Geometry: final body of the model. Coordinates: model frame, mm. Face numbers are marked on the shaded views. Round coordinates to 2 decimals unless told otherwise and drop trailing zeros. Order: outer loops, then holes, each group sorted by start corner. A loop starts at its lowest first (then second) coordinate and runs counter-clockwise, first axis right, second up. Notation, with made-up numbers: (54, 56.5) -> (65, 56.5) arc R7 ccw to (65, 63.5) -> close; hole circle Ø6 at (54, -2). An arc over 180 degrees is marked (long way). Put each result on its own line as item: value.
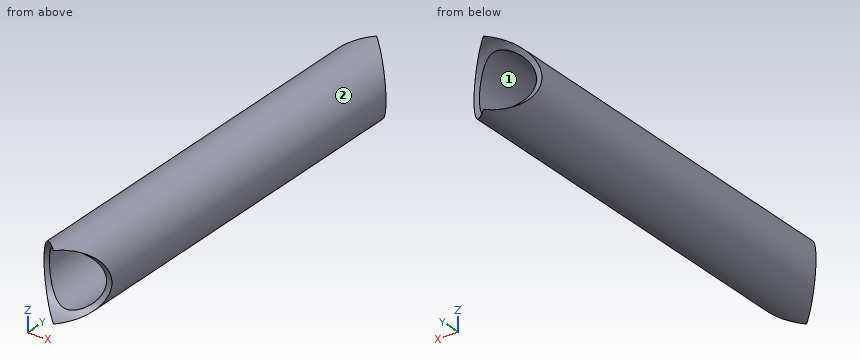
Solid Edge part; units mm, degrees
sketch "Sketch1" plane through (0, 0, 0) normal (0, 0, 1) x (1, 0, 0)
  line L0 (0, 0) -> (0, 164)
sketch "Sketch2" plane through (0, 0, 0) normal (0, -1, 0) x (1, 0, 0)
  circle A0 centre (0, 0) radius 12.5
sweep "SweptProtrusion_1" add profiles "Sketch2" path "Sketch1"
shell "Thinwall_1" thickness 2 removed faces 2 at (-8.0833, 0, 8.5833) at (-8.0833, 164, 8.5833)
sketch "Sketch3" plane through (0, 0, 0) normal (1, 0, 0) x (0, 1, 0)
  circle A0 centre (0, 0) radius 12.5
  circle A1 centre (164, 0) radius 12.5
extrude "Cutout1" cut sketch "Sketch3" along normal through all and the other way through all
properties material "Stainless steel"
1. Draft query along X for the marked faces 1 and 2. Return one class per face: +X half, -X half, draft (parallel to the pull), parting line (faces both ways), or undercut.
Ans:
face 1: undercut
face 2: parting line
2. Contact query for flat-ended pins moving along their axis: P1, Ø2, axis at y = 81, z = 4, coming from the -X side; P2, Ø5, axis at x = -6, y = 57, coming from the -Z side; P3, Ø3, axis at y = 21, z = -7, coming from the -X side (3 decimals). Output: stop coordinate, or through.
Ans:
P1: x = -12.13
P2: z = -12
P3: x = -11.225
3. Cut plane B-B on z = 0. Return loops of the section in (x, y), and give its area (3 significant figures).
Ans:
outline: (-12.5, 12.5) -> (-10.5, 12.5) -> (-10.5, 151.5) -> (-12.5, 151.5) -> close; (10.5, 12.5) -> (12.5, 12.5) -> (12.5, 151.5) -> (10.5, 151.5) -> close
area: 556 mm²
4. Material intervals for probe 1 along Z at (x, y) = (0, 139.5); probe 2 along Z at (x, y) = (-3.75, 148.5), sorted ascending.
Ans:
probe 1: -12.5 to -10.5, 10.5 to 12.5
probe 2: -11.92 to -9.81, 9.81 to 11.92
5. Cut plane A-A on x = 0. Return loops of the section in (y, z), and give its area (3 significant figures).
Ans:
outline: (0, -12.5) -> (164, -12.5) arc R12.5 cw to (157.22, -10.5) -> (6.78, -10.5) arc R12.5 cw to start; (0, 12.5) arc R12.5 cw to (6.78, 10.5) -> (157.22, 10.5) arc R12.5 cw to (164, 12.5) -> close
area: 619 mm²
6. Cut plane C-C on y = 148.5. Return loops of the section in (x, z).
Ans:
outline: circle Ø25 at (0, 0); hole circle Ø21 at (0, 0)
